Autodesk Inventor part; units mm, degrees
ref_plane "YZ Plane" through (0, 0, 0) normal (1, 0, 0) x (0, 1, 0)
ref_plane "XZ Plane" through (0, 0, 0) normal (0, 1, 0) x (-1, 0, 0)
ref_plane "XY Plane" through (0, 0, 0) normal (0, 0, 1) x (1, 0, 0)
sketch "Sketch1" plane through (0, 0, 0) normal (0, 0, 1) x (1, 0, 0)
  line L0 (0, 25.4) -> (-25.4, 0) construction
  line L1 (-25.4, 0) -> (0, -25.4) construction
  line L2 (0, -25.4) -> (25.4, 0) construction
  line L3 (25.4, 0) -> (0, 25.4) construction
  line L4 (0, 25.4) -> (0, -25.4) construction
  line L5 (-25.4, 0) -> (25.4, 0) construction
  line L6 (-28.2284, 2.8284) -> (-2.8284, 28.2284)
  line L7 (2.8284, 28.2284) -> (28.2284, 2.8284)
  line L8 (28.2284, -2.8284) -> (2.8284, -28.2284)
  line L9 (-2.8284, -28.2284) -> (-28.2284, -2.8284)
  arc A0 (2.8284, 28.2284) -> (-2.8284, 28.2284) centre (0, 25.4) ccw
  arc A1 (28.2284, -2.8284) -> (28.2284, 2.8284) centre (25.4, 0) ccw
  arc A2 (-2.8284, -28.2284) -> (2.8284, -28.2284) centre (0, -25.4) ccw
  arc A3 (-28.2284, 2.8284) -> (-28.2284, -2.8284) centre (-25.4, 0) ccw
  circle A4 centre (0, 0) radius 10.0263 construction
  circle A5 centre (0, 0) radius 14.0263
  dimension "d0" = 4
  dimension "d1" = 4
  dimension "d2" = 25.4
  dimension "d22" = 20.0526
  dimension "d23" = 4
extrude "Extrusion1" add sketch "Sketch1" along normal mid plane 10
extrude "Extrusion2" add sketch "Sketch1" along normal mid plane 3 contours A5
sketch "Sketch2" plane through (0, 0, 5) normal (0, 0, 1) x (1, 0, 0)
  arc A0 (28.2284, -2.8284) -> (28.2284, 2.8284) centre (25.4, 0) ccw
  arc A1 (2.8284, 28.2284) -> (-2.8284, 28.2284) centre (0, 25.4) ccw
  arc A2 (-28.2284, 2.8284) -> (-28.2284, -2.8284) centre (-25.4, 0) ccw
  arc A3 (-2.8284, -28.2284) -> (2.8284, -28.2284) centre (0, -25.4) ccw
  point P0 (0, 0)
hole "Hole1" at (0, 25.4, 5) at (-25.4, 0, 5) at (0, -25.4, 5) at (25.4, 0, 5) at (0, 0, 5) direction (0, 0, -1) diameter 3.4 end through all
sketch "Sketch3" plane through (0, 0, -5) normal (0, 0, -1) x (-1, 0, 0)
  circle A0 centre (0, 0) radius 14.0263 construction
  arc A1 (2.8284, 28.2284) -> (-2.8284, 28.2284) centre (0, 25.4) ccw construction
  line L0 (-28.2284, 2.8284) -> (-2.8284, 28.2284) construction
  circle A2 centre (-8.8388, 22.218) radius 4
  line L1 (0, 0) -> (0, 25.4) construction
  circle A3 centre (8.8388, 22.218) radius 4
  dimension "d26" = 8.5
  dimension "d27" = 8
extrude "Extrusion3" cut sketch "Sketch3" against normal through all
fillet "Fillet1" radius 2 4 edges at (6.0104, 25.0464, 0) (11.6673, 19.3896, 0) (-6.0104, 25.0464, 0) (-11.6673, 19.3896, 0)
equation "\"d22\" = 2 * LengthM"
properties part number "MatingPlates"
Build history of the part. All positions in model axes, mm. A direction names the side the tool comes from. Give positions to 0.01 mm unless a question says otherwise; leave off trailing zeros. Order: outer loops, then holes, each group sorted by start corner. A loop starts at its lowest first (then second) coordinate and runs counter-clockwise, first axis right, second up. Notation, with made-up numbers: M 66.25,-28.75 L 76.25,-28.75 A10 cw 76.25,-15.75 Z; hole C 14.5,70 d10. An arc over 180 degrees is marked long. Write item = value, one per line. Start each with the question number.
(1) Probe L1, parallel to Y at x = 0, z = -1.75; L2, parallel to X at y = -0.5, z = 1.25; L3, parallel to X at y = 0, z = 0.75. List the from-to ranges inside material, lowest first. Write a range as [from, to].
(2) Which spindle directions (+Z, -Z, +X, -X, +Y, -Y) get a long thin tool onto all of the face, cutting with end or side? Do faces 5 (the flat face through (3, 0, 1.5)), 6 (the flat face through (20.426, 10.631, -0.07)), 7 (the cylindrical face through (-3, 13.7, -3.3)). Say none if no direction does.
(3) Pin check, flat tips, straight feed: pin 1 Ø6 at (x, z) = (11, -2.5) entering from -Y; pin 2 Ø22.5 at (x, y) = (0, 0) entering from +Z; pin 3 Ø1.5 at (y, z) = (18.5, 4) entering from -X. Stop position of each tip, or through.
(4) Slice it at C-C on y = -25.4. Write the cut outline in (x, z).
(5) Slice it at A-A on y = 0. Write the cut outline in (x, z).
(6) Two-plate mould, pull along Y, no slides. Class faces 1 (the cylindrical face through (-29.4, 0, -0.1)), 2 (the cylindrical face through (0, 29.4, -0.1)), 3 (the cylindrical face through (-6, 19.4, -0.1)), 4 (the flat face through (0, -15, -5)): released by +Y, released by -Y, zero draft, split by the parting line, or undercut.
Responses:
q1.L1 = [-29.4, -27.1], [-23.7, -14.03], [14.03, 23.7], [27.1, 29.4]
q1.L2 = [-29.37, -27.02], [-23.78, -1.62], [1.62, 23.78], [27.02, 29.37]
q1.L3 = [-29.4, -27.1], [-23.7, -1.7], [1.7, 23.7], [27.1, 29.4]
q2.face_5 = +Z
q2.face_6 = +Z, -Z, +X, +Y
q2.face_7 = -Z
q3.pin_1 = -23.06
q3.pin_2 = 1.5
q3.pin_3 = -13.31
q4.outline = M -5.66,-5 L -1.7,-5 L -1.7,5 L -5.66,5 Z; M 1.7,-5 L 5.66,-5 L 5.66,5 L 1.7,5 Z
q5.outline = M -29.4,-5 L -27.1,-5 L -27.1,5 L -29.4,5 Z; M -23.7,-5 L -14.03,-5 L -14.03,-1.5 L -1.7,-1.5 L -1.7,1.5 L -14.03,1.5 L -14.03,5 L -23.7,5 Z; M 1.7,-1.5 L 14.03,-1.5 L 14.03,-5 L 23.7,-5 L 23.7,5 L 14.03,5 L 14.03,1.5 L 1.7,1.5 Z; M 27.1,-5 L 29.4,-5 L 29.4,5 L 27.1,5 Z
q6.face_1 = split by the parting line
q6.face_2 = released by +Y
q6.face_3 = undercut
q6.face_4 = zero draft
